from build123d import *

# Parameters (mm, degrees)
F0_W     = 1524
F0_H     = 1219.2
F1_DEPTH = 50.8
F2_T     = -4.7625
F4_R     = 355.553582
F5_DEPTH = 25.4


with BuildPart() as f1:
    # F0 (on Top) → F1 (new body)
    with BuildSketch(Plane.XY):
        Rectangle(F0_W, F0_H)
    extrude(amount=F1_DEPTH)

    # F2
    f2_openings = [f1.faces().sort_by_distance(p)[0] for p in [
        (0, 0, 50.8),
    ]]
    offset(amount=F2_T, openings=f2_openings)

    # F4 (on face) → F5 (cut)
    with BuildSketch(Plane.XY.offset(4.7625)):
        Circle(F4_R)
    extrude(amount=-F5_DEPTH, mode=Mode.SUBTRACT)


solid = f1.part
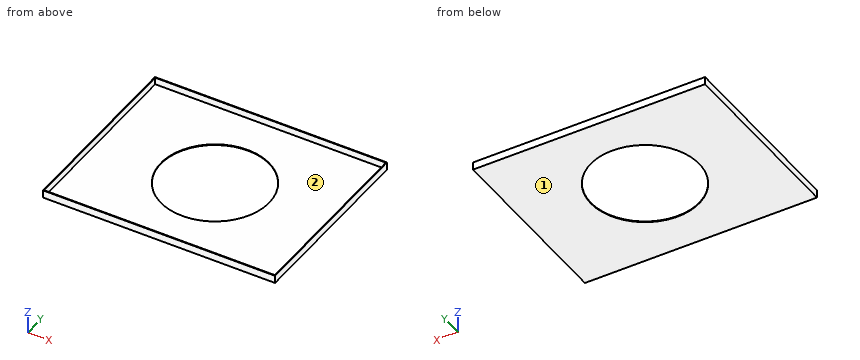
Verification items for the finished model (mm, model axes). Face numbers are marked on the shaded views. Coordinates: 2 decimals unless noted, no trailing zeros. Loops run counter-clockwise (first coordinate to the right, second up) from the corner with the lowest first, then second, coordinate; pieces in that order, holes last. Notation, with made-up numbers: (35, 41) -> (58, 41) arc R19 ccw to (58, 75) -> close; hole circle Ø2 at (28.5, 59.5). An arc over 180 degrees is marked (long way). Answer as a JSON object with one key per item and string values. Group by question number.
Item 1: Sectioned sample at A-A on y = 0. Record the boundary of the cut face in (x, z).
Item 2: Mould release check, pull along Y, two halves, no side actions. Record for the marked faces 1 and 2: +Y half, -Y half, draft (parallel to the pull), parting line (faces both ways), or undercut.
Item 3: Sectioned sample at C-C on z = 21. Record the boundary of the cut face in (x, y), plus the area to 3 significant figures.
Item 4: Sectioned sample at B-B on x = 0. Record the boundary of the cut face in (y, z).
Item 5: Sectioned sample at D-D on x = -374.5. Record the boundary of the cut face in (y, z), plus the area to 3 significant figures.
Item 6: Depth check by flat-ended pin: pin 1 (12 mm diameter, centred on x = 230, y = -425, fed in from +Z). Enter the tip coordinate at first touch or a pass-through.
Item 7: Scan lines: probe 1 along Y at (x, z) = (255, 12.5); probe 2 along Y at (x, z) = (0, 1.3); probe 3 along X at (y, z) = (-82, 26.5). Record each from-to range of solid material in increasing order.
Evaluation:
{
 "1": {"outline": "(-762, 0) -> (-355.55, 0) -> (-355.55, 4.76) -> (-757.24, 4.76) -> (-757.24, 50.8) -> (-762, 50.8) -> close; (355.55, 0) -> (762, 0) -> (762, 50.8) -> (757.24, 50.8) -> (757.24, 4.76) -> (355.55, 4.76) -> close"},
 "2": {"face 1": "draft", "face 2": "undercut"},
 "3": {"outline": "(-762, -609.6) -> (762, -609.6) -> (762, 609.6) -> (-762, 609.6) -> close; hole (-757.24, -604.84) -> (757.24, -604.84) -> (757.24, 604.84) -> (-757.24, 604.84) -> close", "area": "26,000 mm²"},
 "4": {"outline": "(-609.6, 0) -> (-355.55, 0) -> (-355.55, 4.76) -> (-604.84, 4.76) -> (-604.84, 50.8) -> (-609.6, 50.8) -> close; (355.55, 0) -> (609.6, 0) -> (609.6, 50.8) -> (604.84, 50.8) -> (604.84, 4.76) -> (355.55, 4.76) -> close"},
 "5": {"outline": "(-609.6, 0) -> (609.6, 0) -> (609.6, 50.8) -> (604.84, 50.8) -> (604.84, 4.76) -> (-604.84, 4.76) -> (-604.84, 50.8) -> (-609.6, 50.8) -> close", "area": "6,240 mm²"},
 "6": {"pin 1": "stops at z = 4.76"},
 "7": {"probe 1": "y = -609.6 to -604.84, 604.84 to 609.6", "probe 2": "y = -609.6 to -355.55, 355.55 to 609.6", "probe 3": "x = -762 to -757.24, 757.24 to 762"}
}
